Autodesk Inventor part; units mm, degrees
ref_plane "YZ Plane" through (0, 0, 0) normal (1, 0, 0) x (0, 1, 0)
ref_plane "XZ Plane" through (0, 0, 0) normal (0, 1, 0) x (-1, 0, 0)
ref_plane "XY Plane" through (0, 0, 0) normal (0, 0, 1) x (1, 0, 0)
sketch "Sketch1" plane through (0, 0, 0) normal (0, 1, 0) x (-1, 0, 0)
  circle A0 centre (0, 0) radius 60
  dimension "d0" = 120
extrude "Extrusion1" add sketch "Sketch1" along normal blind 50
sketch "Sketch2" plane through (0, 50, 0) normal (0, 1, 0) x (1, 0, 0)
  circle A0 centre (0, 0) radius 50
  dimension "d3" = 100
extrude "Extrusion2" cut sketch "Sketch2" against normal blind 10
fillet "Fillet1" radius 10 1 edges at (-50, 40, 0)
fillet "Fillet2" radius 30 1 edges at (60, 0, 0)
sketch "Sketch3" plane through (0, 0, 0) normal (1, 0, 0) x (0, 1, 0)
  point P0 (0, 0)
properties part number "cylinder_head"
Can you work these out from the model? Positions are in its coordinate system, mm. Round coordinates to 2 decimals unless told otherwise and drop trailing zeros. Loops run counter-clockwise (first coordinate to the right, second up) from the corner with the lowest first, then second, coordinate; pieces in that order, holes last. Notation, with made-up numbers: (2.5, 44.25) - (45.5, 44.25) arc R34 cw to (45.5, 74.25) - close; hole circle Ø2 at (46, 71). An arc over 180 degrees is marked (long way). Answer in a Markdown table with one row per item. Add a question column.
Q1. For pin 1 Ø1.5 at (x, z) = (-1.5, 6.5) entering from +Y; pin 2 Ø2 at (x, y) = (-30, 22.5) entering from +Z; pin 3 Ø8 at (x, y) = (7, 16.5) entering from -Z, each with a flat end and sliding along its axis, tell me the tip position at first contact or that it passes through.
Q2. I need wall thicknesses on L1, parallel to Y at x = -3, z = 3; L2, parallel to Z at x = -42.5, y = 45; L3, parallel to X at y = 15, z = -19. Which ranges of each line are inside material? Lowest first, please.
Q3. We'd pull the mould along X, two halves only. Please class faces 1 (the cylindrical face through (59.94, 39.86, -2.64)), 2 (the flat face through (-1, 40, -1)), 3 (the flat face through (0, 0, 0)): pulls with the +X half, pulls with the -X half, needs draft (parallel to the pull), parting line crosses it, or undercut.
Q4. I want a section at A-A on y = 32.5. List the corners of the cut face in (x, z) for me, and give its area (3 significant figures).
A:
| question | item | result |
|---|---|---|
| 1 | pin 1 | y = 40 |
| 1 | pin 2 | z = 51.5 |
| 1 | pin 3 | z = -58.11 |
| 2 | L1 | 0 to 40 |
| 2 | L2 | -42.35 to -23.7, 23.7 to 42.35 |
| 2 | L3 | -52.66 to 52.66 |
| 3 | face 1 | parting line crosses it |
| 3 | face 2 | undercut |
| 3 | face 3 | needs draft |
| 4 | outline | circle Ø120 at (0, 0) |
| 4 | area | 11,300 mm^2 |
